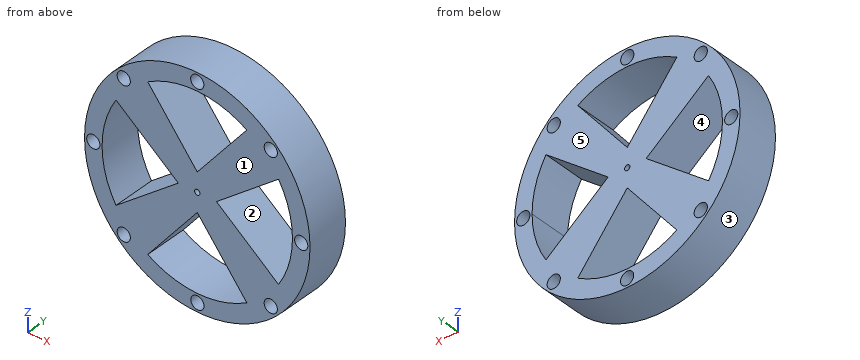
from build123d import *

# Parameters (mm, degrees)
F0_R     = 67.691
F0_R_2   = 3.96875
F0_R_3   = 1.6002
F1_DEPTH = 25.4


with BuildPart() as f1:
    # F0 (on Front) → F1 (new body)
    with BuildSketch(Plane.XZ):
        Circle(F0_R)
        with Locations((-44.1379588351, -44.1379588351)):
            Circle(F0_R_2, mode=Mode.SUBTRACT)
        with Locations((0.085850288, -62.4204405388)):
            Circle(F0_R_2, mode=Mode.SUBTRACT)
        with Locations((44.1379588351, -44.1379588351)):
            Circle(F0_R_2, mode=Mode.SUBTRACT)
        with BuildLine():
            ThreePointArc((-48.797581084, -29.747581084), (-57.15, 0), (-48.797581084, 29.747581084))
            ThreePointArc((-48.797581084, 29.747581084), (-40.4111525448, 40.4111525448), (-29.747581084, 48.797581084))
            ThreePointArc((-29.747581084, 48.797581084), (0, 57.15), (29.747581084, 48.797581084))
            ThreePointArc((29.747581084, 48.797581084), (40.4111525448, 40.4111525448), (48.797581084, 29.747581084))
            ThreePointArc((48.797581084, 29.747581084), (55.0222875704, 15.4489601762), (57.15, 0))
            ThreePointArc((57.15, 0), (55.0222875704, -15.4489601762), (48.797581084, -29.747581084))
            ThreePointArc((48.797581084, -29.747581084), (40.4111525448, -40.4111525448), (29.747581084, -48.797581084))
            ThreePointArc((29.747581084, -48.797581084), (0, -57.15), (-29.747581084, -48.797581084))
            ThreePointArc((-29.747581084, -48.797581084), (-40.4111525448, -40.4111525448), (-48.797581084, -29.747581084))
        make_face(mode=Mode.SUBTRACT)
        with Locations((-62.4204890377, 0.0179510779)):
            Circle(F0_R_2, mode=Mode.SUBTRACT)
        with Locations((-44.1379588351, 44.1379588351)):
            Circle(F0_R_2, mode=Mode.SUBTRACT)
        with Locations((62.420497432, 0.0178410081)):
            Circle(F0_R_2, mode=Mode.SUBTRACT)
        with Locations((0, 62.4205)):
            Circle(F0_R_2, mode=Mode.SUBTRACT)
        with Locations((44.1379588351, 44.1379588351)):
            Circle(F0_R_2, mode=Mode.SUBTRACT)
        with BuildLine():
            ThreePointArc((-29.747581084, 48.797581084), (-40.4111525448, 40.4111525448), (-48.797581084, 29.747581084))
            Line((-48.797581084, 29.747581084), (-11.3440947012, 0.0002201395))
            Line((-11.3440947012, 0.0002201395), (-48.797581084, -29.747581084))
            ThreePointArc((-48.797581084, -29.747581084), (-40.4111525448, -40.4111525448), (-29.747581084, -48.797581084))
            Line((-29.747581084, -48.797581084), (0, -11.3939955701))
            Line((0, -11.3939955701), (29.747581084, -48.797581084))
            ThreePointArc((29.747581084, -48.797581084), (40.4111525448, -40.4111525448), (48.797581084, -29.747581084))
            Line((48.797581084, -29.747581084), (11.515794592, 0))
            Line((11.515794592, 0), (48.797581084, 29.747581084))
            ThreePointArc((48.797581084, 29.747581084), (40.4111525448, 40.4111525448), (29.747581084, 48.797581084))
            Line((29.747581084, 48.797581084), (0, 11.4653596026))
            Line((0, 11.4653596026), (-29.747581084, 48.797581084))
        make_face()
        Circle(F0_R_3, mode=Mode.SUBTRACT)
    extrude(amount=F1_DEPTH)


solid = f1.part
Read the model definition and answer for the solid it produces. Units are mm, in the model's axes. Face numbers are marked on the shaded views. A direction names the side the tool comes from. Coordinates: 2 decimals unless noted, no trailing zeros. Write each loop counter-clockwise with the first axis right and the second up, starting at its lowest first coordinate (ties: lowest second). Pieces come first, ordered by that corner, then holes. Notation, with made-up numbers: (-12.75, 88) - (-7.75, 88) arc R16 cw to (-7.75, 114) - close; hole circle Ø2 at (84, 43.25). An arc over 180 degrees is marked (long way). One line per question, with ' | ' between items.
Q1. For the marked faces 4 and 5, determine the directions among +Z, -Z, +X, -X, +Y, -Y from which every point of the face is accessible in a straight line to the end or side of a thin tool.
Result set:
face 4: +Y, -Y | face 5: +Z, -Z, +X, -X, +Y
Q2. Find section B-B, the plane y = -5.25. State how many separate pieces and enclosed holes the cut face has, plus the area to 3 significant figures.
Result set:
separate pieces: 1 | enclosed holes: 13 | area: 8,200 mm^2
Q3. Find section C-C, the plane x = -43.5. Write down the section's boundary in (y, z).
Result set:
outline: (-25.4, -51.86) - (0, -51.86) - (0, -48.06) - (-25.4, -48.06) - close; (-25.4, -40.22) - (0, -40.22) - (0, -25.54) - (-25.4, -25.54) - close; (-25.4, 25.54) - (0, 25.54) - (0, 40.22) - (-25.4, 40.22) - close; (-25.4, 48.06) - (0, 48.06) - (0, 51.86) - (-25.4, 51.86) - close
Q4. Consider L1, parallel to Z at x = 0, y = -10.5; L2, parallel to X at y = -20.25, z = 25; L3, parallel to X at y = -11.5, z = -7. Determine where each line is inside the solid, lowest interval first. Write a range as [from, to].
Result set:
L1: [-67.69, -66.39], [-58.45, -57.15], [-11.39, -1.6], [1.6, 11.47], [57.15, 58.45], [66.39, 67.69] | L2: [-62.91, -51.39], [-42.82, -10.78], [10.78, 42.85], [51.39, 62.91] | L3: [-67.33, -56.72], [-20.16, 20.29], [56.72, 67.33]
Q5. Determine the mould class of the marked faces 1, 2 and 3 for opening direction X: +X half, -X half, draft (parallel to the pull), parting line (faces both ways), or undercut.
Result set:
face 1: draft | face 2: undercut | face 3: parting line
Q6. Each of these flat-tipped pins is pushed along its axis until it touches: P1, Ø3, axis at y = -4.5, z = -47, coming from the -X side; P2, Ø8, axis at y = -17.5, z = 48, coming from the +X side; P3, Ø5, axis at y = -6.5, z = -53, coming from the -X side. Where does it stop, or does it pass through?
Result set:
P1: x = -50.12 | P2: x = 51.44 | P3: x = -45.08
Q7. Find section A-A, the plane z = -22. Write down the section's boundary in (x, y), plus the area to 3 significant figures.
Result set:
outline: (-64.02, -25.4) - (-52.75, -25.4) - (-52.75, 0) - (-64.02, 0) - close; (-39.04, -25.4) - (-8.44, -25.4) - (-8.44, 0) - (-39.04, 0) - close; (8.44, -25.4) - (39.09, -25.4) - (39.09, 0) - (8.44, 0) - close; (52.75, -25.4) - (64.02, -25.4) - (64.02, 0) - (52.75, 0) - close | area: 2,130 mm^2
